Input: part model. Units: mm. Frame: model coordinates. A direction names the side the tool comes from. Round coordinates to 2 decimals unless told otherwise and drop trailing zeros. Loops run counter-clockwise (first coordinate to the right, second up) from the corner with the lowest first, then second, coordinate; pieces in that order, holes last. Notation, with made-up numbers: M -21,23.25 L -13,23.25 A31 cw -13,53.25 Z; hole C -23,13.25 d11. An arc over 180 degrees is marked long. Return JSON: item names as keys, results as strings. Group by question number.
1) Contact query for flat-ended pins moving along their axis: P1, Ø1.8, axis at x = -18, z = 3, coming from the +Y side; P2, Ø1.8, axis at y = 22.5, z = 1.5, coming from the +X side; P3, Ø1.8, axis at x = 22.5, z = 4, coming from the -Y side. Output: stop coordinate, or through.
2) Section A-A (y = 3). Output: boundary loops of the cut face in (x, z), plus the area to 3 significant figures.
3) Section C-C (z = 2.25). Output: boundary loops of the cut face in (x, y), plus the area to 3 significant figures.
4) Material intervals for line 1 (Y direction, x = 39, z = 1.35); line 2 (X direction, y = -14, z = 3.2); line 3 (Y direction, x = -2, z = 3.95), sorted ascending. Write a range as from..to.
5) Access query for faces 1 (the face through (-32.775, 208.608, 2.958)), 2 (the face through (147, 169.611, 3)), 3 (the face through (100, -77, 3)). Directions: +Z, -Z, +X, -X, +Y, -Y. A direction counts if a zero-diameter tool reaches every point of the face in a straight line with its end or side. Return the directions, or none.
6) Section B-B (x = -32.5). Output: boundary loops of the cut face in (y, z).
from build123d import *

# Parameters (mm, degrees)
F0_W     = 150
F0_H     = 200
F1_DEPTH = 6


with BuildPart() as f1:
    # F0 (on Top) → F1 (new body)
    with BuildSketch(Plane.XY):
        Polygon((0, 213.610874), (-50, 213.610874), (-50, -80.389126), (0, -80.389126), (0, -74.389126), (100, -74.389126), (100, -80.389126), (150, -80.389126), (150, -30.389126), (144, -30.389126), (144, 169.610874), (150, 169.610874), (150, 213.610874), (100, 213.610874), (100, 219.610874), (0, 219.610874), align=None)
        with Locations((50, 44.610874)):
            Rectangle(F0_W, F0_H, mode=Mode.SUBTRACT)
        with BuildLine():
            Line((-45, 181.110874), (-45, 196.110874))
            ThreePointArc((-45, 196.110874), (-32.5, 208.610874), (-20, 196.110874))
            Line((-20, 196.110874), (-20, 181.110874))
            ThreePointArc((-20, 181.110874), (-32.5, 168.610874), (-45, 181.110874))
        make_face(mode=Mode.SUBTRACT)
    extrude(amount=F1_DEPTH)


solid = f1.part
Returned:
{
 "1": {"P1": "stops at y = 213.61", "P2": "stops at x = 144", "P3": "stops at y = -74.39"},
 "2": {"outline": "M -50,0 L -25,0 L -25,6 L -50,6 Z; M 125,0 L 144,0 L 144,6 L 125,6 Z", "area": "264 mm^2"},
 "3": {"outline": "M -50,-80.39 L 0,-80.39 L 0,-74.39 L 100,-74.39 L 100,-80.39 L 150,-80.39 L 150,-30.39 L 144,-30.39 L 144,169.61 L 150,169.61 L 150,213.61 L 100,213.61 L 100,219.61 L 0,219.61 L 0,213.61 L -50,213.61 Z; hole M -45,181.11 A12.5 ccw -20,181.11 L -20,196.11 A12.5 ccw -45,196.11 Z; hole M -25,-55.39 L 125,-55.39 L 125,144.61 L -25,144.61 Z", "area": "26,700 mm^2"},
 "4": {"line 1": "y = -74.39..-55.39, 144.61..219.61", "line 2": "x = -50..-25, 125..144", "line 3": "y = -80.39..-55.39, 144.61..213.61"},
 "5": {"face 1": "+Z, -Z", "face 2": "+Z, -Z, +X", "face 3": "+Z, -Z, -Y"},
 "6": {"outline": "M -80.39,0 L 168.61,0 L 168.61,6 L -80.39,6 Z; M 208.61,0 L 213.61,0 L 213.61,6 L 208.61,6 Z"}
}
